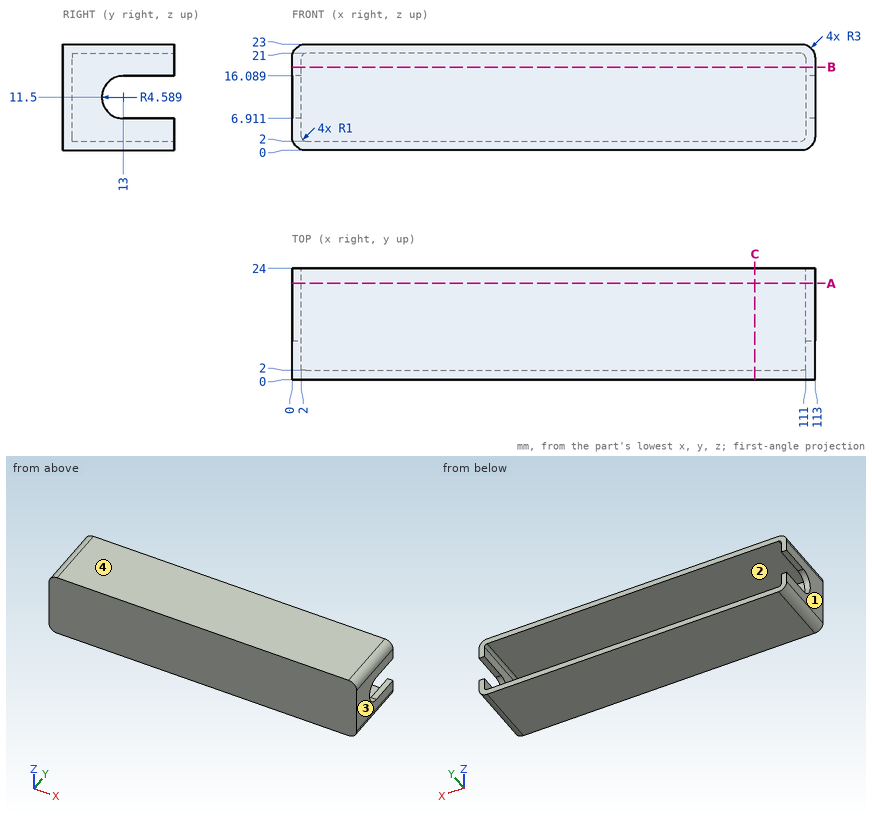
Input: dimensioned drawing with shaded views. Units: mm. Origin: part minimum x, y, z. Round coordinates to 2 decimals unless told otherwise and drop trailing zeros. Order: outer loops, then holes, each group sorted by start corner. A loop starts at its lowest first (then second) coordinate and runs counter-clockwise, first axis right, second up. Notation, with made-up numbers: (-5.5, 49.25) -> (35.5, 49.25) arc R35 cw to (35.5, 81.25) -> close; hole circle Ø5 at (80.5, 27.25). An arc over 180 degrees is marked (long way). Put each result on its own line as item: value. Start each with the question number.
Q1. Section A-A on y = 20.75. Return the cut outline in (x, z).
Q2. Section C-C on x = 100. Return the cut outline in (y, z).
Q3. Pull-direction query (X, two-part tool) for the marked faces 1, 2, 3 and 4; classes: +X half, -X half, draft (parallel to the pull), parting line (faces both ways), or undercut.
Q4. Line query: probe 1 along Z at (x, y) = (29.5, 6); probe 2 along X at (y, z) = (7.25, 11); probe 3 along Y at (x, z) = (44, 5.75). Output: solid intervals per line, ascending.
Q5. Section B-B on z = 18. Return the cut outline in (x, y), and give its area (3 significant figures).
Q6. First-contact query: pin 1 (5 mm diameter, centred on x = 13.5, y = 19.5, fed in from -Z); pin 2 (0.6 mm diameter, centred on x = 1, y = 19.5, fed in from -Z); pin 3 (10 mm diameter, centred on x = 81, z = 12.5, fed in from +Y); pin 4 (1 mm diameter, centred on x = 1, y = 20.5, fed in from +Z). Flat tips, straight axial feed; report the tip coordinate or a pass-through.
Ans:
1. outline: (0, 3) arc R3 ccw to (3, 0) -> (110, 0) arc R3 ccw to (113, 3) -> (113, 6.91) -> (111, 6.91) -> (111, 3) arc R1 cw to (110, 2) -> (3, 2) arc R1 cw to (2, 3) -> (2, 6.91) -> (0, 6.91) -> close; (0, 16.09) -> (2, 16.09) -> (2, 20) arc R1 cw to (3, 21) -> (110, 21) arc R1 cw to (111, 20) -> (111, 16.09) -> (113, 16.09) -> (113, 20) arc R3 ccw to (110, 23) -> (3, 23) arc R3 ccw to (0, 20) -> close
2. outline: (0, 0) -> (24, 0) -> (24, 2) -> (2, 2) -> (2, 21) -> (24, 21) -> (24, 23) -> (0, 23) -> close
3. face 1: -X half
3. face 2: undercut
3. face 3: +X half
3. face 4: draft
4. probe 1: z = 0 to 2, 21 to 23
4. probe 2: x = 0 to 2, 111 to 113
4. probe 3: y = 0 to 2
5. outline: (0, 0) -> (113, 0) -> (113, 24) -> (111, 24) -> (111, 2) -> (2, 2) -> (2, 24) -> (0, 24) -> close
5. area: 314 mm2
6. pin 1: stops at z = 0
6. pin 2: stops at z = 0.53
6. pin 3: stops at y = 2
6. pin 4: stops at z = 22.6
